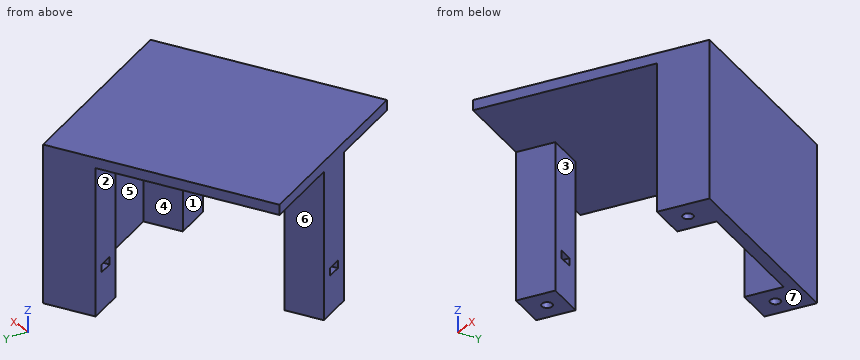
from build123d import *

# Parameters (mm, degrees)
BOX035_W                 = 6
BOX035_H                 = 15
BOX035_DEPTH             = 3
CYLINDER018_R            = 2
CYLINDER018_DEPTH        = 50
BOX_W                    = 15
BOX_H                    = 15
BOX_DEPTH                = 58
BOX038_W                 = 80
BOX038_H                 = 5
BOX038_DEPTH             = 58
BOX039_W                 = 80
BOX039_H                 = 90
BOX039_DEPTH             = 4
CLONE002_PLACEMENT_ANGLE = 120


with BuildPart() as nut_hole:
    # Box035 → Box035 (new body)
    with BuildSketch(Plane(origin=(-8.5, 5, 15), x_dir=(1, 0, 0), z_dir=(0, 0, 1))):
        with Locations((3, 7.5)):
            Rectangle(BOX035_W, BOX035_H)
    extrude(amount=BOX035_DEPTH)


with BuildPart() as cylinder:
    # Cylinder018 → Cylinder018 (new body)
    with BuildSketch(Plane(origin=(-5.5, 12, 0), x_dir=(1, 0, 0), z_dir=(0, 0, 1))):
        Circle(CYLINDER018_R)
    extrude(amount=CYLINDER018_DEPTH)


with BuildPart() as cut:
    # Box → Box (new body)
    with BuildSketch(Plane(origin=(-13, 5, 0), x_dir=(1, 0, 0), z_dir=(0, 0, 1))):
        with Locations((7.5, 7.5)):
            Rectangle(BOX_W, BOX_H)
    extrude(amount=BOX_DEPTH)

    # Cut: cut Cylinder
    add(cylinder.part, mode=Mode.SUBTRACT)


with BuildPart() as cut037:
    # Cut037 base: copy of Cut
    add(cut.part)

    # Cut037: cut Nut hole
    add(nut_hole.part, mode=Mode.SUBTRACT)


with BuildPart() as cut037_1:
    # Cut037 placement: moved
    add(cut037.part.moved(Location((-22, 0, 0))))


with BuildPart() as cut038:
    # Cut038 base: copy of Cut
    add(cut.part)

    # Cut038: cut Nut hole
    add(nut_hole.part, mode=Mode.SUBTRACT)


with BuildPart() as cut038_1:
    # Cut038 placement: moved
    add(cut038.part.moved(Location((43, 0, 0))))


with BuildPart() as extension_supports:
    # Cut039 base: copy of Cut
    add(cut.part)

    # Cut039: cut Nut hole
    add(nut_hole.part, mode=Mode.SUBTRACT)


with BuildPart() as extension_supports_1:
    # Cut039 placement: moved
    add(extension_supports.part.moved(Location((10, 70, 0))))

    # Fusion082: union Cut037, Cut038
    add(cut037_1.part)
    add(cut038_1.part)


with BuildPart() as cube002:
    # Box038 → Box038 (new body)
    with BuildSketch(Plane(origin=(-35, 0, 0), x_dir=(1, 0, 0), z_dir=(0, 0, 1))):
        with Locations((40, 2.5)):
            Rectangle(BOX038_W, BOX038_H)
    extrude(amount=BOX038_DEPTH)


with BuildPart() as clone002:
    # Box039 → Box039 (new body)
    with BuildSketch(Plane(origin=(-35, 0, 58), x_dir=(1, 0, 0), z_dir=(0, 0, 1))):
        with Locations((40, 45)):
            Rectangle(BOX039_W, BOX039_H)
    extrude(amount=BOX039_DEPTH)

    # Fusion081: union Cube002
    add(cube002.part)

    # Fusion084: union Extension supports
    add(extension_supports_1.part)


with BuildPart() as clone002_1:
    # Clone002 placement: moved
    add(clone002.part.moved(Location((122.810889, 195.394192, 0))).rotate(Axis((122.810889, 195.394192, 0), (0, 0, 1)), CLONE002_PLACEMENT_ANGLE))


solid = clone002_1.part
Work out the finished part from the listing and answer in its coordinate system (mm). Face numbers are marked on the shaded views. A direction names the side the tool comes from. Give positions to 0.01 mm unless a question says otherwise; leave off trailing zeros. Order: outer loops, then holes, each group sorted by start corner. A loop starts at its lowest first (then second) coordinate and runs counter-clockwise, first axis right, second up. Notation, with made-up numbers: (51, 1) -> (73, 1) arc R14 ccw to (73, 24) -> close; hole circle Ø3 at (32, -22). An arc over 180 degrees is marked (long way). One line per item, written item: value.
Item 1: Determine the mould class of the marked faces 4, 5, 6 and 7 for opening direction Y: released by +Y, released by -Y, zero draft, split by the parting line, or undercut.
Answer sheet:
face 4: undercut
face 5: undercut
face 6: released by +Y
face 7: zero draft
Item 2: A tool of negligible diameter and unlimited length cuts with its end or side. For the marked faces 1, 2 and 3, from which of +Z, -Z, +X, -X, +Y, -Y can it reach the whole face along a straight path? Write none if from no direction.
Answer sheet:
face 1: -Z, -Y
face 2: -Z, -X, -Y
face 3: -Z, +Y
Item 3: Find section D-D, the plane x = 110. Give the vertices of the cut face in (y, z), plus the area to 3 significant figures.
Answer sheet:
outline: (147.58, 58) -> (207.58, 58) -> (207.58, 0) -> (217.58, 0) -> (217.58, 62) -> (147.58, 62) -> close
area: 860 mm²
Item 4: Find section B-B, the plane z = 46. Give the vertices of the cut face in (x, y), plus the area to 3 significant figures.
Answer sheet:
outline: (38.87, 160.79) -> (46.37, 147.8) -> (59.36, 155.3) -> (51.86, 168.29) -> close; (82.99, 224.37) -> (90.49, 211.37) -> (103.48, 218.87) -> (128.48, 175.57) -> (115.49, 168.07) -> (122.99, 155.08) -> (140.31, 165.08) -> (100.31, 234.37) -> close; hole circle Ø4 at (49.55, 158.29); hole circle Ø4 at (93.67, 221.87); hole circle Ø4 at (126.17, 165.58)
area: 1,040 mm²
Item 5: Find section A-A, the plane z = 53.5. Give the vertices of the cut face in (x, y).
Answer sheet:
outline: (38.87, 160.79) -> (46.37, 147.8) -> (59.36, 155.3) -> (51.86, 168.29) -> close; (82.99, 224.37) -> (90.49, 211.37) -> (103.48, 218.87) -> (128.48, 175.57) -> (115.49, 168.07) -> (122.99, 155.08) -> (140.31, 165.08) -> (100.31, 234.37) -> close
Item 6: Find section C-C, the plane y = 196. Give the vertices of the cut face in (x, z), plus the area to 3 significant figures.
Answer sheet:
outline: (33.86, 58) -> (116.69, 58) -> (116.69, 0) -> (122.46, 0) -> (122.46, 62) -> (33.86, 62) -> close
area: 689 mm²
Item 7: Flat-ended cylindrical pins translate along their axes: P1, Ø5, axis at y = 180.5, z = 47, coming from the -X side; P2, Ø2, axis at y = 221, z = 48.5, coming from the -X side; P3, Ø6, axis at x = 36.5, z = 18, coming from the -Y side. Find the tip coordinate at first contact, or state that the pin passes through.
Answer sheet:
P1: x = 124.19
P2: x = 84.36
P3: y = 159.69
Item 8: Straight lines are drawn through the part: probe 1 along X at (y, z) = (158, 35); probe 2 along Y at (x, z) = (126, 5); probe 3 along Z at (x, y) = (47.5, 179.5). For each, find the intervals that lie inside material, in ascending order.
Answer sheet:
probe 1: 40.48 to 47.57, 51.53 to 57.8, 121.31 to 128.04
probe 2: 156.82 to 163.59, 167.57 to 174.14, 179.87 to 189.87
probe 3: 58 to 62
